Input: dimensioned drawing with shaded views. Units: mm. Origin: part minimum x, y, z. A direction names the side the tool comes from. Round coordinates to 2 decimals unless told otherwise and drop trailing zeros. Loops run counter-clockwise (first coordinate to the right, second up) from the corner with the lowest first, then second, coordinate; pieces in that order, holes last. Notation, with made-up numbers: (82.25, -22.75) - (102.25, -22.75) arc R31 cw to (102.25, 6.25) - close; hole circle Ø3 at (88, 1). An arc over 180 degrees is marked (long way). Write each question's results on one line, items separated by ' | '.
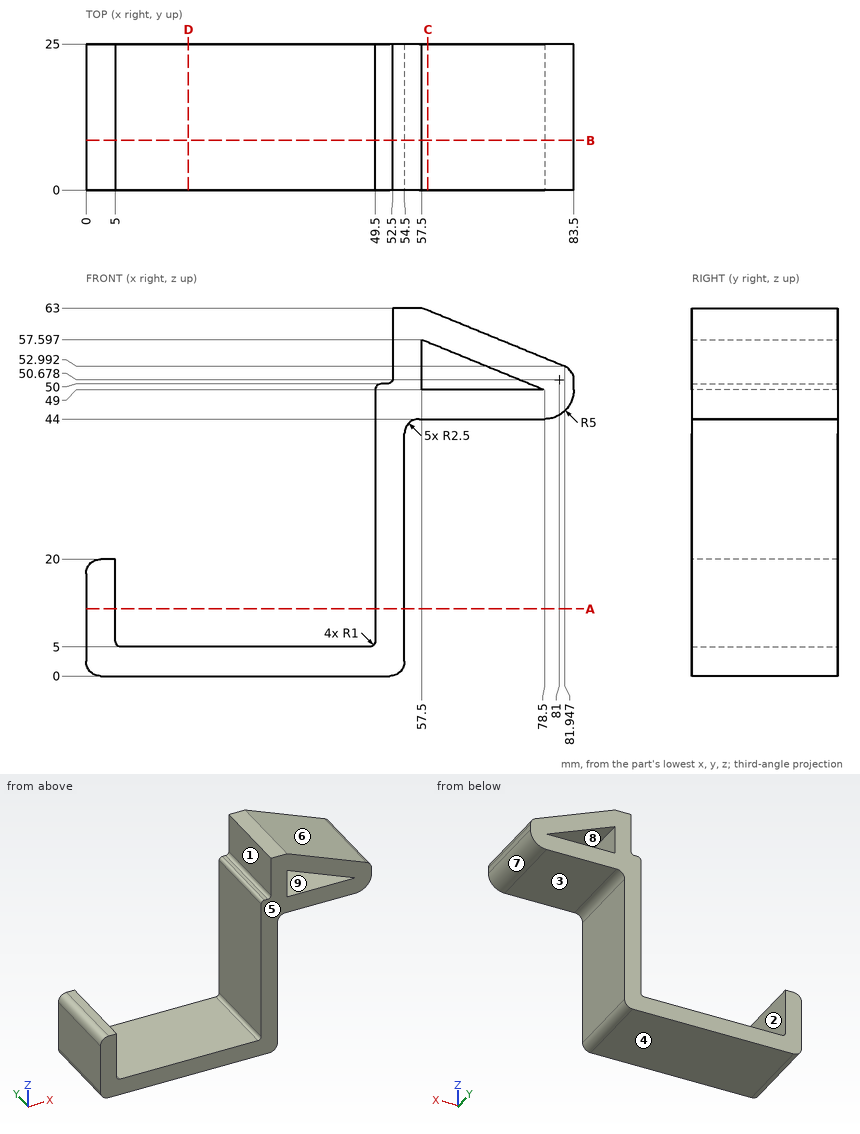
1. Line query: line 1 (X direction, y = 17.25, z = 6); line 2 (Z direction, x = 72, y = 10.25) (1 decimal); line 3 (Z direction, x = 39.5, y = 7.5). Output: solid intervals per line, ascending. Write a range as [from, to].
Answer:
line 1: [0, 5], [49.5, 54.5] | line 2: [44, 49], [51.7, 57.1] | line 3: [0, 5]
2. Section query A-A, the plane z = 11.5. Output: boundary loops of the cut face in (x, y), plus the area to 3 significant figures.
Answer:
outline: (0, 0) - (5, 0) - (5, 25) - (0, 25) - close; (49.5, 0) - (54.5, 0) - (54.5, 25) - (49.5, 25) - close | area: 250 mm^2
3. Mould query, pull axis Z, two halves, no side actions, for the marked faces 6, 7, 8 and 9. Classes: pulls with the +Z half, pulls with the -Z half, needs draft (parallel to the pull), parting line crosses it, or undercut.
Answer:
face 6: pulls with the +Z half | face 7: pulls with the -Z half | face 8: undercut | face 9: undercut
4. Set-up query: the marked faces 1, 2, 3, 4 and 5. Return all of +Z, -Z, +X, -X, +Y, -Y with unobstructed straight access to the full face (end or side cutting, diameter ignored); none if empty.
Answer:
face 1: +Z, -X, +Y, -Y | face 2: +Z, +Y, -Y | face 3: -Z, +X, +Y, -Y | face 4: -Z, +X, -X, +Y, -Y | face 5: +Z, -Z, +X, -X, -Y
5. Section query B-B, the plane y = 8.5. Output: boundary loops of the cut face in (x, z).
Answer:
outline: (0, 2.5) arc R2.5 ccw to (2.5, 0) - (52, 0) arc R2.5 ccw to (54.5, 2.5) - (54.5, 41.5) arc R2.5 cw to (57, 44) - (78.5, 44) arc R5 ccw to (83.5, 49) - (83.5, 50.68) arc R2.5 ccw to (81.95, 52.99) - (57.5, 63) - (52.5, 63) - (52.5, 51) arc R1 cw to (51.5, 50) - (50.5, 50) arc R1 ccw to (49.5, 49) - (49.5, 6) arc R1 cw to (48.5, 5) - (6, 5) arc R1 cw to (5, 6) - (5, 20) - (2.5, 20) arc R2.5 ccw to (0, 17.5) - close; hole (57.5, 49) - (78.5, 49) - (57.5, 57.6) - close
6. Section query D-D, the plane x = 17.5. Output: boundary loops of the cut face in (y, z), plus the area to 3 significant figures.
Answer:
outline: (0, 0) - (25, 0) - (25, 5) - (0, 5) - close | area: 125 mm^2
7. Contact query for flat-ended pins moving along their axis: pin 1 (11 mm diameter, centred on x = 66.5, y = 8, fed in from -Z); pin 2 (13 mm diameter, centred on y = 13, z = 58.5, fed in from -X); pin 3 (1.2 mm diameter, centred on x = 4, y = 18, fed in from +Z). Output: stop coordinate, or through.
Answer:
pin 1: z = 44 | pin 2: x = 52.5 | pin 3: z = 20
8. Section query C-C, the plane x = 58.5. Output: boundary loops of the cut face in (y, z), plus the area to 3 significant figures.
Answer:
outline: (0, 44) - (25, 44) - (25, 49) - (0, 49) - close; (0, 57.19) - (25, 57.19) - (25, 62.59) - (0, 62.59) - close | area: 260 mm^2
